The listing builds one solid part. Answer for the finished solid, in the listing's coordinates (mm). Face numbers are marked on the shaded views. A direction names the side the tool comes from. Give positions to 0.01 mm unless a question says otherwise; leave off trailing zeros. Order: outer loops, then holes, each group sorted by start corner. A loop starts at its lowest first (then second) coordinate and runs counter-clockwise, first axis right, second up. Notation, with made-up numbers: (40, 63.25) - (97, 63.25) arc R31 ccw to (97, 94.25) - close; hole circle Ø5 at (58, -17). An arc over 180 degrees is marked (long way). Answer as CSV lines item,"result". Start each with the question number.
1. Flat-ended cylindrical pins translate along their axes: pin 1 (1.5 mm diameter, centred on y = -16.5, z = -1.5, fed in from -X); pin 2 (5 mm diameter, centred on y = -14.5, z = -1.5, fed in from +X); pin 3 (5 mm diameter, centred on y = -4.5, z = 1.5, fed in from +X). Find the tip coordinate at first contact, or state that the pin passes through.
2. Section B-B on x = 15.5 is taken. Give the vertices of the cut face in (y, z), and give its area (3 significant figures).
3. Which of the six approach directions +Z, -Z, +X, -X, +Y, -Y give full straight-line access (tool end or side, diameter ignored) to the marked faces 1, 2 and 3?
4. Section C-C on y = 4 is taken. Give the vertices of the cut face in (x, z), and give its area (3 significant figures).
5. Section A-A on z = 0 is taken. Give the vertices of the cut face in (x, y).
6. Section D-D on z = 4.25 is taken. Give the vertices of the cut face in (x, y).
7. Consider line 1 along X through (y, z) = (-11, -0.25); line 2 along Y through (x, z) = (12, 0.25); line 3 along X through (y, z) = (-14.5, 4). Determine where each line is inside the solid, lowest interval first. Write a range as [from, to].
from build123d import *

# Parameters (mm, degrees)
SWEEP1_PROFILE_R = 5


with BuildPart() as part:
    # Sweep1: sweep along a path in Sketch1
    with BuildLine(Plane.XY) as sweep1_path:
        Line((-15.72815534, 25), (-6.844660194, 25))
        Line((-6.844660194, 25), (0, 15))
        Line((0, 15), (0, -15))
        Line((0, -15), (6.77184466, -25))
        Line((6.77184466, -25), (17.27184466, -25))
    # Sweep1 profile (on start of the path) → Sweep1 (sweep)
    with BuildSketch(Plane(origin=(-15.72815534, 25, 0), x_dir=(0, 0, 1), z_dir=(1, 0, 0))):
        Circle(SWEEP1_PROFILE_R)
    sweep(path=sweep1_path.line, transition=Transition.RIGHT)


solid = part.part
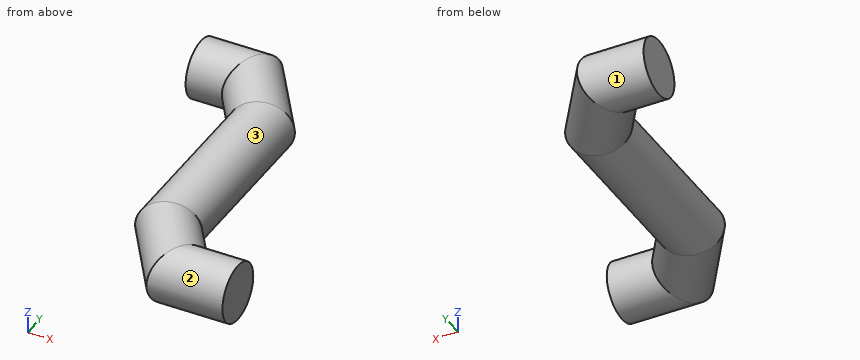
Checks:
1,pin 1,"stops at x = -4.94"
1,pin 2,"stops at x = 7.25"
1,pin 3,"stops at x = 5"
2,outline,"circle Ø10 at (-25, 0)"
2,area,"78.5 mm²"
3,face 1,"-X"
3,face 2,"+X"
3,face 3,"none"
4,outline,"circle Ø10 at (0, 0)"
4,area,"78.5 mm²"
5,outline,"(-15.73, 20) - (-9.48, 20) - (-5, 13.45) - (-5, -16.53) - (4.12, -30) - (17.27, -30) - (17.27, -20) - (9.42, -20) - (5, -13.47) - (5, 16.55) - (-4.21, 30) - (-15.73, 30) - close"
6,outline,"(-15.73, 22.37) - (-8.23, 22.37) - (-2.63, 14.18) - (-2.63, -15.81) - (5.37, -27.63) - (17.27, -27.63) - (17.27, -22.37) - (8.17, -22.37) - (2.63, -14.19) - (2.63, 15.82) - (-5.46, 27.63) - (-15.73, 27.63) - close"
7,line 1,"x = [-4.99, 4.99]"
7,line 2,"y = [-29.99, -20.01]"
7,line 3,"x = [-3, 3.28]"
